```python
from build123d import *

# Parameters (mm, degrees)
F0_W     = 127.9677972198
F0_H     = 50.8497301489
F1_DEPTH = 42.164
F3_W     = 120.4143241048
F3_H     = 43.1107841432
F4_DEPTH = 28.194
F2_W     = 62.752943486
F2_H     = 12.2181459024
F5_DEPTH = 61.468
F6_R     = 4.6974309297
F7_DEPTH = 174.498


with BuildPart() as f1:
    # F0 (on Top) → F1 (new body)
    with BuildSketch(Plane.XY):
        with Locations((-0.2409927547, -9.3987649307)):
            Rectangle(F0_W, F0_H)
    extrude(amount=F1_DEPTH)

    # F3 (on face) → F4 (cut)
    with BuildSketch(Plane.XY.offset(42.164)):
        with Locations((-0.0583641231, -8.8241919875)):
            Rectangle(F3_W, F3_H)
    extrude(amount=-F4_DEPTH, mode=Mode.SUBTRACT)

    # F2 (on face) → F5 (cut)
    with BuildSketch(Plane.XZ.offset(34.8236300051)):
        with Locations((0.2353247255, 36.0549270488)):
            Rectangle(F2_W, F2_H)
    extrude(amount=-F5_DEPTH, mode=Mode.SUBTRACT)

    # F6 (on face) → F7 (cut)
    with BuildSketch(Plane(origin=(-64.2248913646, 0, 0), x_dir=(0, -1, 0), z_dir=(-1, 0, 0))):
        with Locations((6.1297980137, 21.1465246975)):
            Circle(F6_R)
    extrude(amount=-F7_DEPTH, mode=Mode.SUBTRACT)


solid = f1.part
```
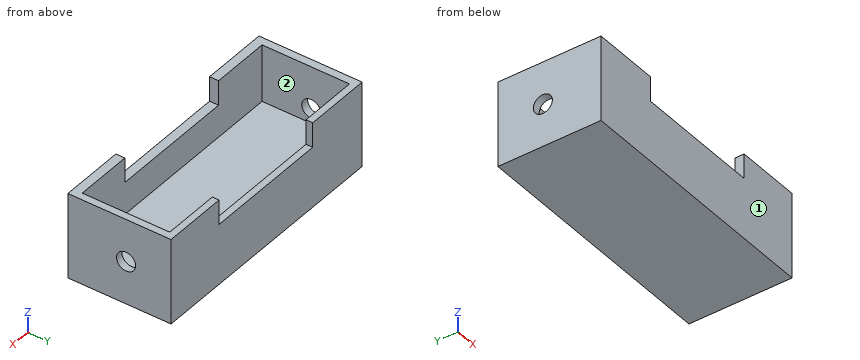
For this review, take the finished solid that the model builds, in its own axes (mm). Face numbers are marked on the shaded views. A direction names the side the tool comes from. Round coordinates to 2 decimals unless told otherwise and drop trailing zeros. Write each loop counter-clockwise with the first axis right and the second up, starting at its lowest first coordinate (ties: lowest second). Pieces come first, ordered by that corner, then holes. Notation, with made-up numbers: (21, 56.5) - (50, 56.5) arc R10 ccw to (50, 66.5) - close; hole circle Ø6 at (12.5, 60.25). An arc over 180 degrees is marked (long way). Use CSV: the item, a comma, the result in double quotes.
1) Clearance check with flat-ended pins moving along their axes: pin 1 Ø1 at (x, y) = (1, 15) entering from +Z; pin 2 Ø8.5 at (y, z) = (-6.13, 21.15) entering from +X; pin 3 Ø1 at (x, y) = (17.5, -27) entering from +Z. State where each tip first meets the part, or that it passes through.
Conclusion:
pin 1,"stops at z = 29.95"
pin 2,"passes through"
pin 3,"stops at z = 13.97"
2) Add section D-D on z = 24.5. Write out the cut boundary in (x, y), and give its area (3 significant figures).
Conclusion:
outline,"(-64.22, -34.82) - (63.74, -34.82) - (63.74, -9.42) - (60.15, -9.42) - (60.15, -30.38) - (-60.27, -30.38) - (-60.27, -9.42) - (-64.22, -9.42) - close; (-64.22, -2.84) - (-60.27, -2.84) - (-60.27, 12.73) - (60.15, 12.73) - (60.15, -2.84) - (63.74, -2.84) - (63.74, 16.03) - (-64.22, 16.03) - close"
area,"1,270 mm^2"
3) Add section B-B on y = -22.5. Write out the cut boundary in (x, z).
Conclusion:
outline,"(-64.22, 0) - (63.74, 0) - (63.74, 42.16) - (60.15, 42.16) - (60.15, 13.97) - (-60.27, 13.97) - (-60.27, 42.16) - (-64.22, 42.16) - close"
4) Add section A-A on z = 32. Write out the cut boundary in (x, y), and give its area (3 significant figures).
Conclusion:
outline,"(-64.22, -34.82) - (-31.14, -34.82) - (-31.14, -30.38) - (-60.27, -30.38) - (-60.27, 12.73) - (-31.14, 12.73) - (-31.14, 16.03) - (-64.22, 16.03) - close; (31.61, -34.82) - (63.74, -34.82) - (63.74, 16.03) - (31.61, 16.03) - (31.61, 12.73) - (60.15, 12.73) - (60.15, -30.38) - (31.61, -30.38) - close"
area,"830 mm^2"
5) Wall thickness on line 1 along X through (y, z) = (-31, 37); line 2 along Y through (x, z) = (-45, 19); line 3 along X through (y, z) = (3, 18): over which ranges is each line inside the solid? List them lowest first. Write a range as from..to.
Conclusion:
line 1,"x = -64.22..-31.14, 31.61..63.74"
line 2,"y = -34.82..-30.38, 12.73..16.03"
line 3,"x = -64.22..-60.27, 60.15..63.74"
6) Add section C-C on x = 3. Write out the cut boundary in (y, z), and give its area (3 significant figures).
Conclusion:
outline,"(-34.82, 0) - (16.03, 0) - (16.03, 29.95) - (12.73, 29.95) - (12.73, 13.97) - (-30.38, 13.97) - (-30.38, 29.95) - (-34.82, 29.95) - close"
area,"834 mm^2"
7) For the marked faces 1 and 2, list the 3-axis set-ups (+Z, -Z, +X, -X, +Y, -Y) from which the entire face can be reached by the end or side of a thin tool; tool diameter is ignored.
Conclusion:
face 1,"+Z, -Z, +X, -X, -Y"
face 2,"+Z"
